```python
from build123d import *

# Parameters (mm, degrees)
SKETCH1_W           = 508
SKETCH1_H           = 165.1
BOSS_EXTRUDE2_DEPTH = 63.5
CUT_EXTRUDE2_DEPTH  = 275.522772279
SHELL1_T            = -6.35
FILLET1_R           = 5
FILLET2_R           = 3.18


with BuildPart() as part:
    # Sketch1 → Boss-Extrude2 (new body)
    with BuildSketch(Plane(origin=(0, 0, 0), x_dir=(0, 0, -1), z_dir=(1, 0, 0))):
        Rectangle(SKETCH1_W, SKETCH1_H)
    extrude(amount=BOSS_EXTRUDE2_DEPTH)

    # Sketch14 → Cut-Extrude2 (cut, through all)
    with BuildSketch(Plane(origin=(63.5, 0, 0), x_dir=(0, 0, -1), z_dir=(1, 0, 0))):
        with BuildLine():
            Line((-153.67, -82.55), (-153.67, -59.9))
            ThreePointArc((-153.67, -59.9), (-133.35, -39.58), (-113.03, -59.9))
            Line((-113.03, -59.9), (-113.03, -82.55))
            ThreePointArc((-113.03, -82.55), (-133.35, -102.87), (-153.67, -82.55))
        make_face()
        with BuildLine():
            Line((-7.62, -82.55), (-7.62, -59.9))
            ThreePointArc((-7.62, -59.9), (12.7, -39.58), (33.02, -59.9))
            Line((33.02, -59.9), (33.02, -82.55))
            ThreePointArc((33.02, -82.55), (12.7, -102.87), (-7.62, -82.55))
        make_face()
        with BuildLine():
            Line((138.43, -82.55), (138.43, -59.9))
            ThreePointArc((138.43, -59.9), (158.75, -39.58), (179.07, -59.9))
            Line((179.07, -59.9), (179.07, -82.55))
            ThreePointArc((179.07, -82.55), (158.75, -102.87), (138.43, -82.55))
        make_face()
    extrude(amount=-CUT_EXTRUDE2_DEPTH, mode=Mode.SUBTRACT)

    # Shell1
    shell1_openings = [part.faces().sort_by_distance(p)[0] for p in [
        (0, 3.74487295, 0.755170832),
    ]]
    offset(amount=SHELL1_T, openings=shell1_openings, kind=Kind.INTERSECTION)

    # Fillet1
    fillet1_edges = [part.edges().sort_by_distance(p)[0] for p in [
        (63.5, 0, 254),
        (63.5, -82.55, 203.835),
        (63.5, -82.55, 60.325),
        (63.5, -82.55, -85.725),
        (63.5, -82.55, -216.535),
        (63.5, -71.225, 153.67),
        (63.5, -71.225, 113.03),
        (63.5, -39.58, 133.35),
        (63.5, -71.225, 7.62),
        (63.5, -71.225, -33.02),
        (63.5, -39.58, -12.7),
        (63.5, -71.225, -138.43),
        (63.5, -71.225, -179.07),
        (63.5, -39.58, -158.75),
        (63.5, 0, -254),
        (63.5, 82.55, 0),
    ]]
    fillet(fillet1_edges, radius=FILLET1_R)

    # Fillet2
    fillet2_edges = [part.edges().sort_by_distance(p)[0] for p in [
        (57.15, -76.2, 60.325),
        (57.15, -76.2, -85.725),
        (57.15, -76.2, -216.535),
        (57.15, 0, -247.65),
        (57.15, 76.2, 0),
        (57.15, 0, 247.65),
        (57.15, -76.2, 203.835),
        (57.15, -68.05, -132.08),
        (57.15, -33.23, -158.75),
        (57.15, -68.05, -185.42),
        (57.15, -68.05, 13.97),
        (57.15, -33.23, -12.7),
        (57.15, -68.05, -39.37),
        (57.15, -68.05, 160.02),
        (57.15, -33.23, 133.35),
        (57.15, -68.05, 106.68),
    ]]
    fillet(fillet2_edges, radius=FILLET2_R)


solid = part.part
```
Read the model definition and answer for the solid it produces. Units are mm, in the model's axes. A direction names the side the tool comes from. Round coordinates to 2 decimals unless told otherwise and drop trailing zeros. Write each loop counter-clockwise with the first axis right and the second up, starting at its lowest first coordinate (ties: lowest second). Pieces come first, ordered by that corner, then holes. Notation, with made-up numbers: M 20,-21 L 41,-21 A26 cw 41,11 Z; hole C 25,56.5 d10. An arc over 180 degrees is marked long. One line per item, written item: value.
Q1. A flat-ended cylindrical pin translates along its axis: pin 1 Ø6 at (y, z) = (-37.5, 18) entering from -X. Find the tip coordinate at first contact, or state that the pin passes through.
Data:
pin 1: x = 57.15
Q2. Straight lines are drawn through the part: line 1 (Y direction, x = 4.5, z = 14.5); line 2 (Z direction, x = 6.5, y = 28); line 3 (X direction, y = 25.5, z = -107.5). For each, find the intervals that lie inside material, in ascending order. Write a range as [from, to].
Data:
line 1: [-82.55, -76.2], [76.2, 82.55]
line 2: [-254, -247.65], [247.65, 254]
line 3: [57.15, 63.5]
Q3. Find section D-D on y = -51. Count the separate pieces of the cut face and the enclosed holes in it, plus the area to 3 significant figures.
Data:
separate pieces: 4
enclosed holes: 0
area: 5,580 mm2
Q4. Find section C-C on z = -158.75. Write down the section's boundary in (x, y).
Data:
outline: M 0,-39.58 L 58.5,-39.58 A5 ccw 63.5,-34.58 L 63.5,77.55 A5 ccw 58.5,82.55 L 0,82.55 L 0,76.2 L 53.97,76.2 A3.18 cw 57.15,73.02 L 57.15,-30.05 A3.18 cw 53.97,-33.23 L 0,-33.23 Z
Q5. Which of the six approach directions +Z, -Z, +X, -X, +Y, -Y give full straight-line access (tool end or side, diameter ignored) to faces 1 (the flat face through (30, -71, 113.03)), 2 (the flat face through (27, -1, 247.65)), 3 (the flat face through (29, -1, -254))?
Data:
face 1: +X, -X, -Y
face 2: -X
face 3: -Z, +X, -X, +Y, -Y
Q6. For a pull along Y with two mould halves and no side action, classify faces 4 (the cylindrical face through (27.363, -33.236, -158.164)), 5 (the flat face through (0, -36, -18)), 6 (the flat face through (29, -82.55, 205)), 7 (the flat face through (29, 82.55, 4)) as +Y half, -Y half, draft (parallel to the pull), parting line (faces both ways), or undercut.
Data:
face 4: undercut
face 5: draft
face 6: -Y half
face 7: +Y half
Q7. Find section B-B on y = 48. Write down the section's boundary in (x, z).
Data:
outline: M 0,-254 L 58.5,-254 A5 ccw 63.5,-249 L 63.5,249 A5 ccw 58.5,254 L 0,254 L 0,247.65 L 53.97,247.65 A3.18 cw 57.15,244.47 L 57.15,-244.47 A3.18 cw 53.97,-247.65 L 0,-247.65 Z
